The figure shows three views and two pictorial views of one solid part (mm, origin at its lowest corner). Answer the questions. Coordinates: 2 decimals unless noted, no trailing zeros. Loops run counter-clockwise (first coordinate to the right, second up) from the corner with the lowest first, then second, coordinate; pieces in that order, holes last. Notation, with made-up numbers: M -14.75,70.5 L 28.25,70.5 A25 cw 28.25,94.5 Z; hole C -36,66 d11. An arc over 180 degrees is marked long. Return JSON: item names as keys, results as strings. Group by question number.
1. Section B-B (x = 2.3) is taken. Write down the section's boundary in (y, z).
2. Section C-C (z = 1.15) is taken. Write down the section's boundary in (x, y) (3 decimals), then the cut area to 3 significant figures.
3. Section A-A (y = 1.25) is taken. Write down the section's boundary in (x, z) (3 decimals).
4. The mould has two halves that part along X. Classify the marked faces 1, 2, 3 and 4: pulls with the +X half, pulls with the -X half, needs draft (parallel to the pull), parting line crosses it, or undercut.
5. Section D-D (y = 3.25) is taken. Write down the section's boundary in (x, z).
6. Straight lines are drawn through the part: L1, parallel to X at y = 5.75, z = 2.25 (3 decimals); L2, parallel to Z at x = 3.25, y = 1.75 (3 decimals); L3, parallel to Y at x = 2.65, z = 2.85. For each, find the intervals that lie inside material, in ascending order. Write a range as from..to.
7. Given P1, Ø1, axis at x = 1.5, y = 6.5, coming from the -Z side (3 decimals), flat-ended and moving along its own axis, determine where the tip first touches the part or whether it passes through.
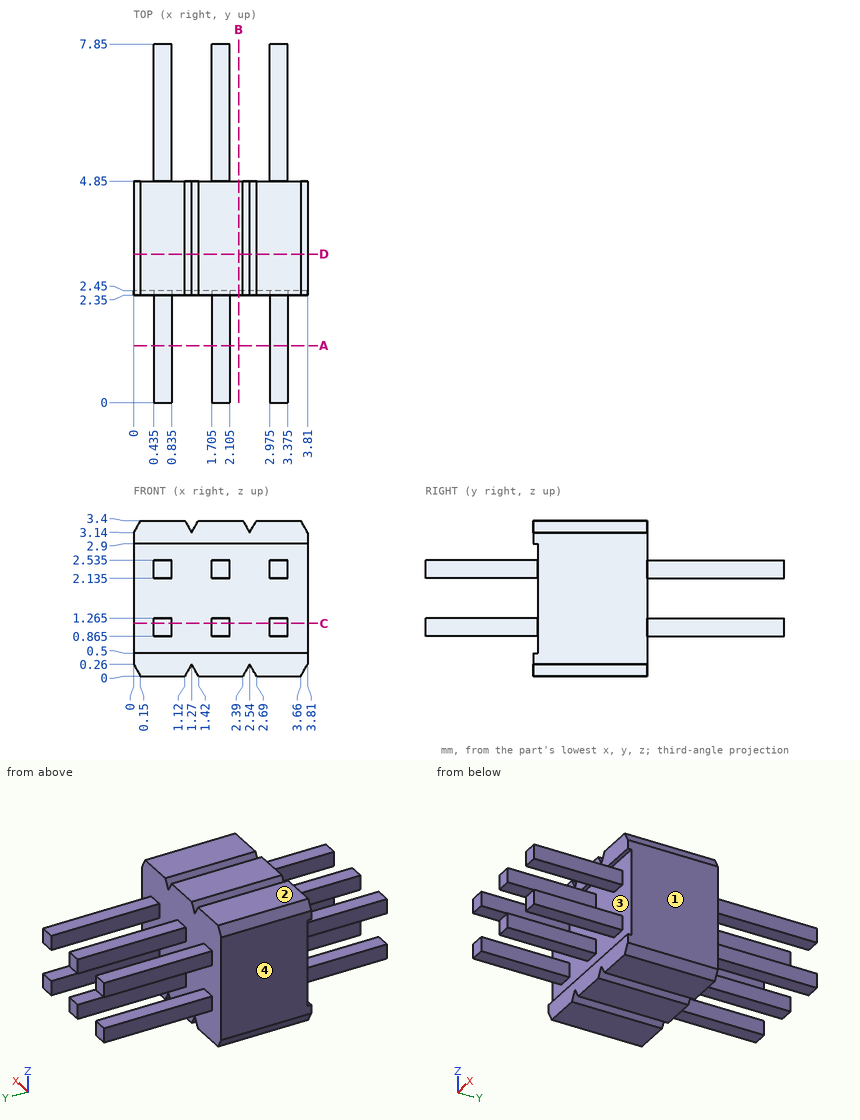
Worked out:
{
 "1": {"outline": "M 2.35,0 L 4.85,0 L 4.85,3.4 L 2.35,3.4 L 2.35,2.9 L 2.45,2.9 L 2.45,0.5 L 2.35,0.5 Z"},
 "2": {"outline": "M 0,2.45 L 0.435,2.45 L 0.435,0 L 0.835,0 L 0.835,2.45 L 1.705,2.45 L 1.705,0 L 2.105,0 L 2.105,2.45 L 2.975,2.45 L 2.975,0 L 3.375,0 L 3.375,2.45 L 3.81,2.45 L 3.81,4.85 L 3.375,4.85 L 3.375,7.85 L 2.975,7.85 L 2.975,4.85 L 2.105,4.85 L 2.105,7.85 L 1.705,7.85 L 1.705,4.85 L 0.835,4.85 L 0.835,7.85 L 0.435,7.85 L 0.435,4.85 L 0,4.85 Z", "area": "15.7 mm^2"},
 "3": {"outline": "M 0.435,0.865 L 0.835,0.865 L 0.835,1.265 L 0.435,1.265 Z; M 0.435,2.135 L 0.835,2.135 L 0.835,2.535 L 0.435,2.535 Z; M 1.705,0.865 L 2.105,0.865 L 2.105,1.265 L 1.705,1.265 Z; M 1.705,2.135 L 2.105,2.135 L 2.105,2.535 L 1.705,2.535 Z; M 2.975,0.865 L 3.375,0.865 L 3.375,1.265 L 2.975,1.265 Z; M 2.975,2.135 L 3.375,2.135 L 3.375,2.535 L 2.975,2.535 Z"},
 "4": {"face 1": "pulls with the +X half", "face 2": "needs draft", "face 3": "undercut", "face 4": "pulls with the -X half"},
 "5": {"outline": "M 0,0.26 L 0.15,0 L 1.12,0 L 1.27,0.26 L 1.42,0 L 2.39,0 L 2.54,0.26 L 2.69,0 L 3.66,0 L 3.81,0.26 L 3.81,3.14 L 3.66,3.4 L 2.69,3.4 L 2.54,3.14 L 2.39,3.4 L 1.42,3.4 L 1.27,3.14 L 1.12,3.4 L 0.15,3.4 L 0,3.14 Z"},
 "6": {"L1": "0.435..0.835, 1.705..2.105, 2.975..3.375", "L2": "0.865..1.265, 2.135..2.535", "L3": "2.45..4.85"},
 "7": {"P1": "z = 0.865"}
}
